For this review, take the finished solid that the model builds, in its own axes (mm). A direction names the side the tool comes from. Round coordinates to 2 decimals unless told otherwise and drop trailing zeros. Write each loop counter-clockwise with the first axis right and the second up, starting at its lowest first coordinate (ties: lowest second). Pieces come first, ordered by that corner, then holes. Notation, with made-up numbers: (81.25, 82) -> (138.25, 82) arc R17 ccw to (138.25, 88) -> close; hole circle Ø3 at (54, 20). An arc over 180 degrees is marked (long way). Answer in a Markdown table with one row per item. Add a question column.
```python
from build123d import *

# Parameters (mm, degrees)
SKETCH2_W          = 32.004
SKETCH2_H          = 83.312
SKETCH2_W_2        = 16.002
SKETCH2_H_2        = 41.656
CUT_EXTRUDE1_DEPTH = 4.826


with BuildPart() as part:
    # Sketch1 → Revolve1 (revolve)
    with BuildSketch(Plane.XY):
        Polygon((0, 0), (0, 8.9154), (0.762, 9.6774), (4.0386, 9.6774), (4.8006, 8.9154), (5.5626, 8.9154), (5.5626, 10.414), (12.7254, 10.414), (13.4874, 9.652), (13.4874, 0), align=None)
    revolve(axis=Axis((13.4874, 0, 0), (-1, 0, 0)))

    # Sketch2 → Cut-Extrude1 (cut)
    with BuildSketch(Plane(origin=(13.4874, 0, 0), x_dir=(0, 0, -1), z_dir=(1, 0, 0))):
        Rectangle(SKETCH2_W, SKETCH2_H)
        Rectangle(SKETCH2_W_2, SKETCH2_H_2, mode=Mode.SUBTRACT)
    extrude(amount=-CUT_EXTRUDE1_DEPTH, mode=Mode.SUBTRACT)

    # Sketch3 → Hole1 (revolve, cut)
    with BuildSketch(Plane.ZX):
        Polygon((0, 0), (0, 6.35), (6.35, 6.35), (6.35, 0.254), (6.604, 0), align=None)
    revolve(axis=Axis((-6.445314094, 0, 0), (1, 0, 0)), mode=Mode.SUBTRACT)

    # Sketch5 → Hole2 (revolve, cut)
    with BuildSketch(Plane(origin=(13.4874, 0, 0), x_dir=(0, 0, -1), z_dir=(0, 1, 0))):
        Polygon((0, 0), (0, 13.8684), (1.98374, 13.8684), (1.98374, 0.81026), (2.413, 0.381), (2.413, 0), align=None)
    revolve(axis=Axis((19.617423899, 0, 0), (-1, 0, 0)), mode=Mode.SUBTRACT)

    # Sketch7 → Revolve2 (revolve)
    with BuildSketch(Plane.XY):
        Polygon((4.46379893, 10.329831804), (5.878230735, 8.9154), (6.16559893, 8.9154), (4.66699893, 10.414), (4.46379893, 10.414), align=None)
    revolve(axis=Axis((13.4874, 0, 0), (-1, 0, 0)))


solid = part.part
```
1. We need section B-B (x = 1.75). Write out the cut boundary in (y, z).
2. Tool access review of faces 4 (the cylindrical face through (9.558, -1.967, 0.258)), 5 (the conical face through (13.37, -9.77, -0.13)), 6 (the flat face through (11, 0, 8.001)), 7 (the cylindrical face through (3.26, 6.2, -1.38)), 8 (the flat face through (8.661, 0, -9)): name each direction out of +Z, -Z, +X, -X, +Y, -Y from which nothing blocks a thin tool from reaching the whole face with its end or side.
3. For L1, parallel to Y at x = 3, z = 0; L2, parallel to Y at x = 5, z = 0; L3, parallel to Z at x = 8.5, y = 0, list the stretches that pass through material, from the lowest coordinate up. Write a range as [from, to].
4. We need section A-A (x = 12.25). Write out the cut boundary in (y, z).
5. We need section C-C (x = 8). Write out the cut boundary in (y, z).
6. Clearance check with flat-ended pins moving along their axes: pin 1 Ø1 at (y, z) = (1.5, 4.5) entering from -X; pin 2 Ø1 at (x, z) = (10, 3.5) entering from +Y; pin 3 Ø3 at (x, y) = (10.5, -2.5) entering from +Z. State where each tip first meets the part, or that it passes through.
7. The part is to be moulded in two halves that separate along X. For faces 1 (the flat face through (8.661, 0, 9)), 2 (the cylindrical face through (13.3, 1.468, 1.915)), 3 (the cylindrical face through (5.187, -8.907, -0.392)), say which applies: pulls with the +X half, pulls with the -X half, needs draft (parallel to the pull), parting line crosses it, or undercut.
Response:
| question | item | result |
|---|---|---|
| 1 | outline | circle Ø19.35 at (0, 0); hole circle Ø12.7 at (0, 0) |
| 2 | face 4 | +X, -X |
| 2 | face 5 | +X, -Y |
| 2 | face 6 | +Z, +X, +Y, -Y |
| 2 | face 7 | -X |
| 2 | face 8 | -Z, +X, +Y, -Y |
| 3 | L1 | [-9.68, -6.35], [6.35, 9.68] |
| 3 | L2 | [-10.08, -9.79], [-8.92, -6.35], [6.35, 8.92], [9.79, 10.08] |
| 3 | L3 | [-10.41, -1.98], [1.98, 10.41] |
| 4 | outline | (-6.67, -8) -> (6.67, -8) arc R10.41 ccw to (6.67, 8) -> (-6.67, 8) arc R10.41 ccw to start; hole circle Ø3.97 at (0, 0) |
| 5 | outline | circle Ø20.83 at (0, 0); hole circle Ø3.97 at (0, 0) |
| 6 | pin 1 | x = 6.35 |
| 6 | pin 2 | y = 9.97 |
| 6 | pin 3 | z = 8 |
| 7 | face 1 | pulls with the +X half |
| 7 | face 2 | needs draft |
| 7 | face 3 | undercut |
